Part model, mm, in its own coordinate system. A direction names the side the tool comes from. Coordinates: 2 decimals unless noted, no trailing zeros. Order: outer loops, then holes, each group sorted by start corner. A loop starts at its lowest first (then second) coordinate and runs counter-clockwise, first axis right, second up. Notation, with made-up numbers: M 64.5,12.25 L 92.5,12.25 A11 ccw 92.5,16.25 Z; hole C -40,43 d4. An arc over 180 degrees is marked long. Answer in a Markdown table with one row per item. Add a question column.
from build123d import *

# Parameters (mm, degrees)
BOSS_EXTRUDE2_DEPTH = 4.7
SKETCH4_W           = 3
SKETCH4_H           = 3.5
CUT_EXTRUDE1_DEPTH  = 5


with BuildPart() as part:
    # Sketch3 → Boss-Extrude2 (new body)
    with BuildSketch(Plane.XY):
        Polygon((-3.35, 5), (-3.35, -5), (3.35, -5), (3.35, 5), (6.63, 5), (10.65, 5), (11.65, 5), (11.65, 15), (10.65, 15), (-3.35, 15), align=None)
        with BuildLine():
            Line((10.1, 11), (4.1, 11))
            ThreePointArc((4.1, 11), (7.1, 14), (10.1, 11))
        make_face(mode=Mode.SUBTRACT)
        with BuildLine():
            Line((10.1, 6), (4.1, 6))
            ThreePointArc((4.1, 6), (7.1, 9), (10.1, 6))
        make_face(mode=Mode.SUBTRACT)
    extrude(amount=BOSS_EXTRUDE2_DEPTH)

    # Sketch4 → Cut-Extrude1 (cut)
    with BuildSketch(Plane.ZY.offset(3.35)):
        with Locations((2.35, 7.597247867)):
            Rectangle(SKETCH4_W, SKETCH4_H)
        with Locations((2.35, 12.597247867)):
            Rectangle(SKETCH4_W, SKETCH4_H)
    extrude(amount=-CUT_EXTRUDE1_DEPTH, mode=Mode.SUBTRACT)


solid = part.part
(1) Slice it at B-B (z = 1.8). List the corners of the cut face in (x, y).
(2) Slice it at A-A (x = 7.1). List the corners of the cut face in (y, z), and give its area (3 significant figures).
(3) 3-axis set-ups, long thin cutter, end or side, ignore diameter. For faces 5 (the flat face through (3.35, 0, 2)), 6 (the flat face through (-1, 8, 0.85)), 7 (the cylindrical face through (7, 14, 2)): which of +Z, -Z, +X, -X, +Y, -Y reach the whole face in a straight line?
(4) Drop a flat-ended pin along its axis: P1, Ø0.9, axis at y = 7.5, z = 3, coming from the -X side. Give the stop position or say it passes through.
(5) Pull direction X, two halves, no side cores. Call faces 1 (the flat face through (7, 11, 2)), 2 (the flat face through (1.65, 13, 2)), 3 (the flat face through (7, 6, 2)), 4 (the flat face through (11.65, 10, 2)): pulls with the +X half, pulls with the -X half, needs draft (parallel to the pull), parting line crosses it, or undercut.
(6) Slice it at D-D (x = 5.5). List the corners of the cut face in (y, z), and give its area (3 significant figures).
(7) Slice it at C-C (y = 11.25). List the corners of the cut face in (x, z).
(8) Wall check: line 1 (Y direction, x = 1.5, z = 3.6); line 2 (Z direction, x = 1, y = 9); line 3 (Y direction, x = 7.75, z = 1.45). Give the ranges that are in metal, low to high.
Computed:
| question | item | result |
|---|---|---|
| 1 | outline | M -3.35,-5 L 3.35,-5 L 3.35,5 L 11.65,5 L 11.65,15 L -3.35,15 L -3.35,14.35 L 1.65,14.35 L 1.65,10.85 L -3.35,10.85 L -3.35,9.35 L 1.65,9.35 L 1.65,5.85 L -3.35,5.85 Z; hole M 4.1,6 L 10.1,6 A3 ccw Z; hole M 4.1,11 L 10.1,11 A3 ccw Z |
| 2 | outline | M 5,0 L 6,0 L 6,4.7 L 5,4.7 Z; M 9,0 L 11,0 L 11,4.7 L 9,4.7 Z; M 14,0 L 15,0 L 15,4.7 L 14,4.7 Z |
| 2 | area | 18.8 mm^2 |
| 3 | face 5 | +Z, -Z, +X, -Y |
| 3 | face 6 | -X |
| 3 | face 7 | +Z, -Z |
| 4 | P1 | stops at x = 1.65 |
| 5 | face 1 | undercut |
| 5 | face 2 | pulls with the -X half |
| 5 | face 3 | undercut |
| 5 | face 4 | pulls with the +X half |
| 6 | outline | M 5,0 L 6,0 L 6,4.7 L 5,4.7 Z; M 8.54,0 L 11,0 L 11,4.7 L 8.54,4.7 Z; M 13.54,0 L 15,0 L 15,4.7 L 13.54,4.7 Z |
| 6 | area | 23.1 mm^2 |
| 7 | outline | M -3.35,0 L 4.11,0 L 4.11,4.7 L -3.35,4.7 L -3.35,3.85 L 1.65,3.85 L 1.65,0.85 L -3.35,0.85 Z; M 10.09,0 L 11.65,0 L 11.65,4.7 L 10.09,4.7 Z |
| 8 | line 1 | y = -5 to 5.85, 9.35 to 10.85, 14.35 to 15 |
| 8 | line 2 | z = 0 to 0.85, 3.85 to 4.7 |
| 8 | line 3 | y = 5 to 6, 8.93 to 11, 13.93 to 15 |
